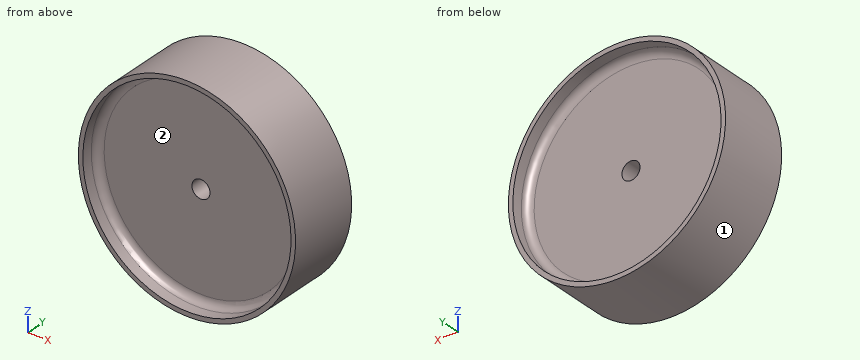
from build123d import *

# Parameters (mm, degrees)
SKETCH1_R           = 38.1
SKETCH1_R_2         = 3.175
BOSS_EXTRUDE1_DEPTH = 12.7
SKETCH2_R           = 38.1
SKETCH2_R_2         = 36.5125
BOSS_EXTRUDE2_DEPTH = 6.35
BOSS_EXTRUDE3_START = 6.35
SKETCH3_R           = 38.1
SKETCH3_R_2         = 36.5125
BOSS_EXTRUDE3_DEPTH = 6.35
FILLET1_R           = 2.54


with BuildPart() as part:
    # Sketch1 → Boss-Extrude1 (new body)
    with BuildSketch(Plane(origin=(0, 0, 0), x_dir=(1, 0, 0), z_dir=(0, 1, 0))):
        with Locations(Location((0, 0, 0), (0, 0, 270))):
            Circle(SKETCH1_R)
        with Locations(Location((0, 0, 0), (0, 0, 270))):
            Circle(SKETCH1_R_2, mode=Mode.SUBTRACT)
    extrude(amount=BOSS_EXTRUDE1_DEPTH)

    # Sketch2 → Boss-Extrude2 (add)
    with BuildSketch(Plane(origin=(0, 12.7, 0), x_dir=(1, 0, 0), z_dir=(0, 1, 0))):
        with Locations(Location((0, 0, 0), (0, 0, 270))):
            Circle(SKETCH2_R)
        with Locations(Location((0, 0, 0), (0, 0, 270))):
            Circle(SKETCH2_R_2, mode=Mode.SUBTRACT)
    extrude(amount=BOSS_EXTRUDE2_DEPTH)

    # Sketch3 → Boss-Extrude3 (add)
    with BuildSketch(Plane.XZ.offset(BOSS_EXTRUDE3_START)):
        with Locations(Location((0, 0, 0), (0, 0, 270))):
            Circle(SKETCH3_R)
        with Locations(Location((0, 0, 0), (0, 0, 90))):
            Circle(SKETCH3_R_2, mode=Mode.SUBTRACT)
    extrude(amount=-BOSS_EXTRUDE3_DEPTH)

    # Fillet1
    fillet1_edges = [part.edges().sort_by_distance(p)[0] for p in [
        (0, 0, -36.5125),
        (0, 12.7, -36.5125),
    ]]
    fillet(fillet1_edges, radius=FILLET1_R)


solid = part.part
Source: CAD feature listing. Evaluate the final solid. Frame: model axes, mm. Face numbers are marked on the shaded views. Coordinates: 2 decimals unless noted, no trailing zeros. Order: outer loops, then holes, each group sorted by start corner. A loop starts at its lowest first (then second) coordinate and runs counter-clockwise, first axis right, second up. Notation, with made-up numbers: M 27,50 L 85,50 A6 ccw 85,59 Z; hole C 11.5,57.25 d7. An arc over 180 degrees is marked long. Write each question's results on one line, items separated by ' | '. Start each with the question number.
Item 1: Line query: probe 1 along X at (y, z) = (18, 0); probe 2 along X at (y, z) = (7.5, 0) (3 decimals); probe 3 along Y at (x, z) = (-20.5, -1.5). Output: solid intervals per line, ascending.
Item 2: Cut plane C-C (y = 1). Return loops of the section in (x, z) (3 decimals).
Item 3: First-contact query: pin 1 Ø6 at (x, y) = (24, 3.5) entering from -Z; pin 2 Ø4 at (x, z) = (0, 0) entering from +Y; pin 3 Ø1.5 at (x, z) = (26, 5.5) entering from -Y; pin 4 Ø1.5 at (x, y) = (-14, 13.5) entering from +Z. Flat tips, straight axial feed; report the tip coordinate or a pass-through.
Item 4: Draft query along X for the marked faces 1 and 2. Return one class per face: pulls with the +X half, pulls with the -X half, needs draft (parallel to the pull), parting line crosses it, or undercut.
Checked values:
1) probe 1: x = -38.1 to -36.51, 36.51 to 38.1 | probe 2: x = -38.1 to -3.175, 3.175 to 38.1 | probe 3: y = 0 to 12.7
2) outline: C 0,0 d76.2; hole C 0,0 d6.35
3) pin 1: stops at z = -31.79 | pin 2: passes through | pin 3: stops at y = 0 | pin 4: stops at z = 35.72
4) face 1: parting line crosses it | face 2: undercut
